Autodesk Inventor part; units mm, degrees
ref_plane "YZ Plane" through (0, 0, 0) normal (1, 0, 0) x (0, 1, 0)
ref_plane "XY Plane" through (0, 0, 0) normal (0, 0, 1) x (1, 0, 0)
sketch "Sketch1" plane through (0, 0, 0) normal (0, 0, 1) x (1, 0, 0)
  line L0 (0, 0) -> (70, 0)
  line L1 (0, 6) -> (0, 0)
  line L2 (50, 6) -> (50, 5)
  line L3 (50, 5) -> (70, 5)
  line L4 (70, 5) -> (70, 0)
  line L5 (50, 6) -> (0, 6)
  line L6 (0, 6) -> (0, 5)
  line L7 (0, 5) -> (-20, 5)
  line L8 (-20, 5) -> (-20, 0)
  line L9 (-20, 0) -> (0, 0)
  dimension "d10" = 1
  dimension "d11" = 20
  dimension "d12" = 5
  dimension "d16" = 20
  dimension "d17" = 5
  dimension "d18" = 50
revolve "Revolution1" add sketch "Sketch1" angle 360 about axis through (0, 0, 0) along (1, 0, 0)
thread "Thread2"
ref_plane "Work Plane1" through (25, 0, 0) normal (1, 0, 0) x (0, 0, -1)
chamfer "Chamfer2" distance 1 angle 45 2 edges at (70, -5, 0) (-20, -5, 0)
properties part number "Rocker Base Shaft"
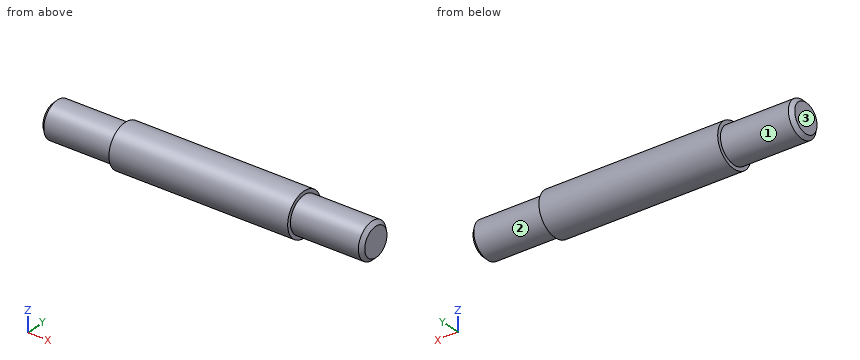
Read the model definition and answer for the solid it produces. Units are mm, in the model's axes. Face numbers are marked on the shaded views. A direction names the side the tool comes from. Coordinates: 2 decimals unless noted, no trailing zeros. Write each loop counter-clockwise with the first axis right and the second up, starting at its lowest first coordinate (ties: lowest second). Pieces come first, ordered by that corner, then holes. Notation, with made-up numbers: (14.25, 1.5) -> (39.25, 1.5) arc R7 cw to (39.25, 6.5) -> close; hole circle Ø5 at (34, 34.25). An arc over 180 degrees is marked (long way). Answer as a JSON object with one key per item and string values.
Q1. Flat-ended cylindrical pins translate along their axes: pin 1 Ø1 at (x, y) = (16.5, 1.5) entering from -Z; pin 2 Ø6 at (x, z) = (2, 3.5) entering from +Y; pin 3 Ø3 at (x, y) = (17, 4.5) entering from -Z. Find the tip coordinate at first contact, or state that the pin passes through.
The answers:
{"pin 1": "stops at z = -5.92", "pin 2": "stops at y = 5.98", "pin 3": "stops at z = -5.2"}
Q2. The part is cut by section D-D on x = 20.5. Give the vertices of the cut face in (y, z).
The answers:
{"outline": "circle Ø12 at (0, 0)"}
Q3. The part is cut by section A-A on z = 0. Give the vertices of the cut face in (x, y), then the cut area to 3 significant figures.
The answers:
{"outline": "(-20, -4) -> (-19, -5) -> (0, -5) -> (0, -6) -> (50, -6) -> (50, -5) -> (69, -5) -> (70, -4) -> (70, 4) -> (69, 5) -> (50, 5) -> (50, 6) -> (0, 6) -> (0, 5) -> (-19, 5) -> (-20, 4) -> close", "area": "998 mm2"}
Q4. The part is cut by section C-C on x = -7. Give the vertices of the cut face in (y, z).
The answers:
{"outline": "circle Ø10 at (0, 0)"}
Q5. Consider line 1 (Y direction, x = -3, z = 0.25); line 2 (X direction, y = 2.25, z = 5); line 3 (Y direction, x = 25.5, z = -2). Determine where each line is inside the solid, lowest interval first. Write a range as [from, to].
The answers:
{"line 1": "y = [-4.99, 4.99]", "line 2": "x = [0, 50]", "line 3": "y = [-5.66, 5.66]"}
Q6. A tool of negligible diameter and unlimited length cuts with its end or side. For the marked faces 1, 2 and 3, from which of +Z, -Z, +X, -X, +Y, -Y can it reach the whole face along a straight path? Write none if from no direction.
The answers:
{"face 1": "-X", "face 2": "+X", "face 3": "+Z, -Z, -X, +Y, -Y"}
